```python
from build123d import *

# Parameters (mm, degrees)
SKETCH1_W           = 7.6
SKETCH1_H           = 10.5
BOSS_EXTRUDE1_DEPTH = 2.65
SKETCH2_W           = 0.5
SKETCH2_H           = 1.4
BOSS_EXTRUDE2_DEPTH = 1.4
SKETCH4_W           = 0.5
SKETCH4_H           = 1.4
BOSS_EXTRUDE3_DEPTH = 1.4


with BuildPart() as part:
    # Sketch1 → Boss-Extrude1 (new body)
    with BuildSketch(Plane(origin=(0, 0, 0), x_dir=(1, 0, 0), z_dir=(0, 1, 0))):
        Rectangle(SKETCH1_W, SKETCH1_H)
    extrude(amount=BOSS_EXTRUDE1_DEPTH)

    # Sketch2 → Boss-Extrude2 (add)
    with BuildSketch(Plane.ZY.offset(3.8)):
        with Locations((-4.871874673, 0.7)):
            Rectangle(SKETCH2_W, SKETCH2_H)
        with Locations((-3.601874673, 0.7)):
            Rectangle(SKETCH2_W, SKETCH2_H)
        with Locations((-2.331874673, 0.7)):
            Rectangle(SKETCH2_W, SKETCH2_H)
        with Locations((-1.061874673, 0.7)):
            Rectangle(SKETCH2_W, SKETCH2_H)
        with Locations((0.208125327, 0.7)):
            Rectangle(SKETCH2_W, SKETCH2_H)
        with Locations((1.478125327, 0.7)):
            Rectangle(SKETCH2_W, SKETCH2_H)
        with Locations((2.748125327, 0.7)):
            Rectangle(SKETCH2_W, SKETCH2_H)
        with Locations((4.018125327, 0.7)):
            Rectangle(SKETCH2_W, SKETCH2_H)
    extrude(amount=BOSS_EXTRUDE2_DEPTH)

    # Sketch4 → Boss-Extrude3 (add)
    with BuildSketch(Plane(origin=(3.8, 0, 0), x_dir=(0, 0, -1), z_dir=(1, 0, 0))):
        with Locations((-4.626381769, 0.7)):
            Rectangle(SKETCH4_W, SKETCH4_H)
        with Locations((-3.356381769, 0.7)):
            Rectangle(SKETCH4_W, SKETCH4_H)
        with Locations((-2.086381769, 0.7)):
            Rectangle(SKETCH4_W, SKETCH4_H)
        with Locations((2.086381769, 0.7)):
            Rectangle(SKETCH4_W, SKETCH4_H)
        with Locations((3.356381769, 0.7)):
            Rectangle(SKETCH4_W, SKETCH4_H)
        with Locations((4.626381769, 0.7)):
            Rectangle(SKETCH4_W, SKETCH4_H)
    extrude(amount=BOSS_EXTRUDE3_DEPTH)


solid = part.part
```
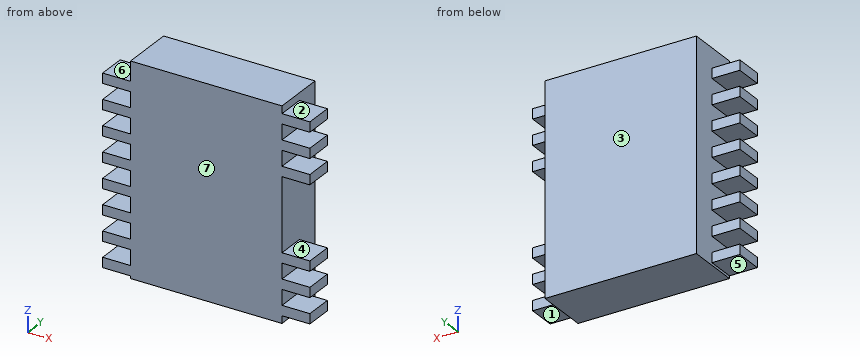
Check sheet for the modelled part. Datum: model origin and axes. Units: mm. Face numbers are marked on the shaded views. A direction names the side the tool comes from. Coordinates: 2 decimals unless noted, no trailing zeros. Write each loop counter-clockwise with the first axis right and the second up, starting at its lowest first coordinate (ties: lowest second). Pieces come first, ordered by that corner, then holes. Notation, with made-up numbers: M 19.5,4.25 L 45.5,4.25 A24 cw 45.5,20.25 Z; hole C 83,31 d6. An arc over 180 degrees is marked long. Use one line per item in the form item = value.
Item 1: Sectioned sample at D-D, the plane y = 2.15. Record the cut outline in (x, z).
Answer below:
outline = M -3.8,-5.25 L 3.8,-5.25 L 3.8,5.25 L -3.8,5.25 Z
Item 2: Gauge pin test, flat ends, axial feed: pin 1 Ø0.7 at (x, y) = (4.5, 0.5) entering from -Z; pin 2 Ø1.1 at (x, y) = (-4.5, 0.5) entering from +Z; pin 3 Ø1.1 at (x, y) = (4.5, 0.5) entering from +Z. Record the tip position at first contact, or that the pin passes through.
Answer below:
pin_1 = -4.88
pin_2 = 4.27
pin_3 = 4.88
Item 3: Set-up check for the marked faces 1, 2 and 3: record each of +Z, -Z, +X, -X, +Y, -Y from which the full face is reachable in a straight line by a thin tool's end or side.
Answer below:
face_1 = -Z, +X, +Y, -Y
face_2 = +Z, +X, +Y, -Y
face_3 = +Z, -Z, +X, -X, +Y
Item 4: Sectioned sample at B-B, the plane x = 4.5. Record the cut outline in (y, z).
Answer below:
outline = M 0,-4.88 L 1.4,-4.88 L 1.4,-4.38 L 0,-4.38 Z; M 0,-3.61 L 1.4,-3.61 L 1.4,-3.11 L 0,-3.11 Z; M 0,-2.34 L 1.4,-2.34 L 1.4,-1.84 L 0,-1.84 Z; M 0,1.84 L 1.4,1.84 L 1.4,2.34 L 0,2.34 Z; M 0,3.11 L 1.4,3.11 L 1.4,3.61 L 0,3.61 Z; M 0,4.38 L 1.4,4.38 L 1.4,4.88 L 0,4.88 Z
Item 5: Material ranges on L1, parallel to X at y = 0.95, z = 0.25; L2, parallel to X at y = 0.75, z = 4.5; L3, parallel to Y at x = -4.5, z = 2.75, recorded low to high. Write a range as from..to.
Answer below:
L1 = -5.2..3.8
L2 = -3.8..5.2
L3 = 0..1.4
Item 6: Release check for a two-part mould opening along Z. For the marked faces 4, 5, 6 and 7 record: pulls with the +Z half, pulls with the -Z half, needs draft (parallel to the pull), parting line crosses it, or undercut.
Answer below:
face_4 = undercut
face_5 = pulls with the -Z half
face_6 = pulls with the +Z half
face_7 = needs draft
Item 7: Sectioned sample at A-A, the plane x = -4. State how many separate pieces and enclosed holes the cut face has, and give its area (3 significant figures).
Answer below:
separate_pieces = 8
enclosed_holes = 0
area = 5.60 mm^2
Item 8: Sectioned sample at C-C, the plane z = 2. Record the cut outline in (x, y), and give its area (3 significant figures).
Answer below:
outline = M -3.8,0 L 5.2,0 L 5.2,1.4 L 3.8,1.4 L 3.8,2.65 L -3.8,2.65 Z
area = 22.1 mm^2
